For this review, use the dimensioned drawing (mm, ordinates from the lowest corner) and the shaded views. A direction names the side the tool comes from. Coordinates: 2 decimals unless noted, no trailing zeros. Write each loop counter-clockwise with the first axis right and the second up, starting at its lowest first coordinate (ties: lowest second). Pieces come first, ordered by that corner, then holes. Notation, with made-up numbers: M -30.75,32 L -5.75,32 A14 ccw -5.75,56 Z; hole C -1.75,14 d5. An arc over 180 degrees is marked long. One line per question, with ' | ' between items.
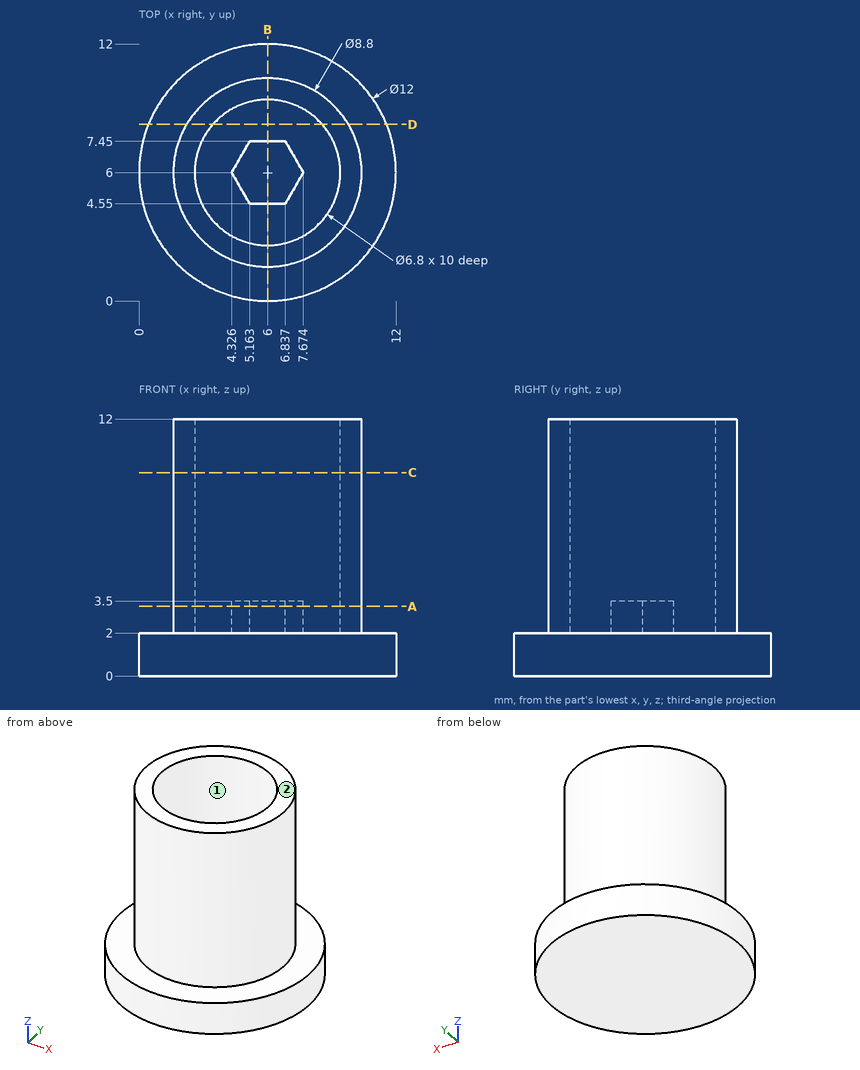
1) We need section C-C on z = 9.5. State the section outline as (x, y) points, then the cut area to 3 significant figures.
Responses:
outline: C 6,6 d8.8; hole C 6,6 d6.8 | area: 24.5 mm^2
2) Insertion check: pin 1 Ø1.2 at (x, z) = (6, 3) entering from +Y; pin 2 Ø4 at (y, z) = (10.5, 7.5) entering from -X; pin 3 Ø1.5 at (x, y) = (6, 5.5) entering from +Z. Each pin has a flat end and moves straight along its axis. Give the tip position at first contact, or say it passes through.
Responses:
pin 1: y = 10.4 | pin 2: x = 2.38 | pin 3: z = 3.5
3) We need section D-D on y = 8.25. State the section outline as (x, z) points.
Responses:
outline: M 0.44,0 L 11.56,0 L 11.56,2 L 9.78,2 L 9.78,12 L 8.55,12 L 8.55,2 L 3.45,2 L 3.45,12 L 2.22,12 L 2.22,2 L 0.44,2 Z
4) Machinability: for the marked faces 1 and 2, which of the approach directions +Z, -Z, +X, -X, +Y, -Y give a long, thin tool a straight path to every point of the face, cutting with its end or side? Answer none if there is none.
Responses:
face 1: +Z | face 2: +Z, +X, -X, +Y, -Y
5) To check wall thickness, follow line 1 along Y through (x, z) = (6, 7.5); line 2 along Z through (x, y) = (10, 8.5); line 3 along Y through (x, z) = (6.75, 4.5) (1 decimal). State the ranges of each line that lie inside material, in increasing order. Write a range as [from, to].
Responses:
line 1: [1.6, 2.6], [9.4, 10.4] | line 2: [0, 2] | line 3: [1.7, 2.7], [9.3, 10.3]
6) We need section B-B on x = 6. State the section outline as (y, z) points.
Responses:
outline: M 0,0 L 12,0 L 12,2 L 10.4,2 L 10.4,12 L 9.4,12 L 9.4,2 L 7.45,2 L 7.45,3.5 L 4.55,3.5 L 4.55,2 L 2.6,2 L 2.6,12 L 1.6,12 L 1.6,2 L 0,2 Z
7) We need section A-A on z = 3.25. State the section outline as (x, y) points.
Responses:
outline: C 6,6 d8.8; M 4.33,6 L 5.16,4.55 L 6.84,4.55 L 7.67,6 L 6.84,7.45 L 5.16,7.45 Z; hole C 6,6 d6.8
